Input: part model. Units: mm. Frame: model coordinates. A direction names the side the tool comes from. Round coordinates to 2 decimals unless told otherwise and drop trailing zeros. Loops run counter-clockwise (first coordinate to the right, second up) from the corner with the lowest first, then second, coordinate; pieces in that order, holes last.
1) Access query for faces 1 (the face through (1, 0.5, -3)), 2 (the face through (-3.787, 3.359, -0.841)), 3 (the face through (0.03, 1.11, 14.75)). Directions: +Z, -Z, +X, -X, +Y, -Y. A direction counts if a zero-diameter tool reaches every point of the face in a straight line with its end or side. Return the directions, or none.
2) First-contact query: pin 1 (5.5 mm diameter, centred on x = 1.5, z = 5.5, fed in from +Y); pin 2 (0.9 mm diameter, centred on x = 0, z = 15.5, fed in from -Y); pin 3 (4.5 mm diameter, centred on x = 0, z = 0, fed in from +Y); pin 4 (2 mm diameter, centred on x = 2, z = 7, fed in from +Y). Flat tips, straight axial feed; report the tip coordinate or a pass-through.
3) Section D-D, the plane y = 3.55. Return loops of the section in (x, z), and give its area (3 significant figures).
4) Section B-B, the plane z = 0. Return loops of the section in (x, y).
5) Ray query, line 1 along X through (y, z) = (0.4, 0.5); line 2 along X through (y, z) = (0.2, -0.75); line 3 along X through (y, z) = (1.3, 19). Return the intervals inside material, ascending.
6) Section A-A, the plane y = 1.9. Return loops of the section in (x, z).
7) Section C-C, the plane x = 0. State how many separate pieces and enclosed holes the cut face has, and give its area (3 significant figures).
8) Draft query along Z for faces 4 (the face through (-3, 4.5, 0)), 5 (the face through (0, 1.1, 20.6)), 6 (the face through (0.03, 1.11, 7.75)). Return one class per face: pulls with the +Z half, pulls with the -Z half, needs draft (parallel to the pull), parting line crosses it, or undercut.
from build123d import *

# Parameters (mm, degrees)
SKETCH1_R           = 2.5
SKETCH1_R_2         = 0.75
BOSS_EXTRUDE1_DEPTH = 2.25
SKETCH2_R           = 3.879501895
SKETCH2_R_2         = 2.5
BOSS_EXTRUDE2_DEPTH = 2.25
SKETCH3_R           = 2.5
SKETCH3_R_2         = 2.008527967
BOSS_EXTRUDE3_DEPTH = 1
SKETCH4_R           = 3.8
SKETCH4_R_2         = 3
CUT_EXTRUDE1_DEPTH  = 0.5
CUT_EXTRUDE2_DEPTH  = 22.766258291


with BuildPart() as part:
    # Sketch1 → Boss-Extrude1 (new body)
    with BuildSketch(Plane(origin=(0, 0, 0), x_dir=(1, 0, 0), z_dir=(0, 1, 0))):
        with BuildLine():
            Line((-1.6, 19), (-3.75, 3.885550154))
            ThreePointArc((-3.75, 3.885550154), (-5.4, 0), (-3.75, -3.885550154))
            Line((-3.75, -3.885550154), (-1.6, -19))
            ThreePointArc((-1.6, -19), (0, -20.6), (1.6, -19))
            Line((1.6, -19), (3.75, -3.885550154))
            ThreePointArc((3.75, -3.885550154), (5.4, 0), (3.75, 3.885550154))
            Line((3.75, 3.885550154), (1.6, 19))
            ThreePointArc((1.6, 19), (0, 20.6), (-1.6, 19))
        make_face()
        with Locations(Location((0, 0, 0), (0, 0, 270))):
            Circle(SKETCH1_R, mode=Mode.SUBTRACT)
        with Locations(Location((0, -19, 0), (0, 0, 270))):
            Circle(SKETCH1_R_2, mode=Mode.SUBTRACT)
        with Locations(Location((0, 19, 0), (0, 0, 270))):
            Circle(SKETCH1_R_2, mode=Mode.SUBTRACT)
        with Locations(Location((0, 15.5, 0), (0, 0, 270))):
            Circle(SKETCH1_R_2, mode=Mode.SUBTRACT)
        with Locations(Location((0, 12, 0), (0, 0, 270))):
            Circle(SKETCH1_R_2, mode=Mode.SUBTRACT)
        with Locations(Location((0, 8.5, 0), (0, 0, 270))):
            Circle(SKETCH1_R_2, mode=Mode.SUBTRACT)
        with Locations(Location((0, -15.5, 0), (0, 0, 270))):
            Circle(SKETCH1_R_2, mode=Mode.SUBTRACT)
        with Locations(Location((0, -12, 0), (0, 0, 270))):
            Circle(SKETCH1_R_2, mode=Mode.SUBTRACT)
        with Locations(Location((0, -8.5, 0), (0, 0, 270))):
            Circle(SKETCH1_R_2, mode=Mode.SUBTRACT)
    extrude(amount=BOSS_EXTRUDE1_DEPTH)

    # Sketch2 → Boss-Extrude2 (add)
    with BuildSketch(Plane(origin=(0, 2.25, 0), x_dir=(1, 0, 0), z_dir=(0, 1, 0))):
        with Locations(Location((0, 0, 0), (0, 0, 270))):
            Circle(SKETCH2_R)
        with Locations(Location((0, 0, 0), (0, 0, 270))):
            Circle(SKETCH2_R_2, mode=Mode.SUBTRACT)
    extrude(amount=BOSS_EXTRUDE2_DEPTH)

    # Sketch3 → Boss-Extrude3 (add)
    with BuildSketch(Plane.XZ):
        with Locations(Location((0, 0, 0), (0, 0, 270))):
            Circle(SKETCH3_R)
        with Locations(Location((0, 0, 0), (0, 0, 270))):
            Circle(SKETCH3_R_2, mode=Mode.SUBTRACT)
    extrude(amount=-BOSS_EXTRUDE3_DEPTH)

    # Sketch4 → Cut-Extrude1 (cut)
    with BuildSketch(Plane.XZ):
        with Locations(Location((0, 0, 0), (0, 0, 270))):
            Circle(SKETCH4_R)
        with Locations(Location((0, 0, 0), (0, 0, 270))):
            Circle(SKETCH4_R_2, mode=Mode.SUBTRACT)
    extrude(amount=-CUT_EXTRUDE1_DEPTH, mode=Mode.SUBTRACT)

    # Sketch5 → Cut-Extrude2 (cut, through all)
    with BuildSketch(Plane.XZ):
        with BuildLine():
            Line((-3.75, -3.885550154), (-1.6, -19))
            ThreePointArc((-1.6, -19), (0, -20.6), (1.6, -19))
            Line((1.6, -19), (3.75, -3.885550154))
            ThreePointArc((3.75, -3.885550154), (0, -5.4), (-3.75, -3.885550154))
        make_face()
    extrude(amount=-CUT_EXTRUDE2_DEPTH, mode=Mode.SUBTRACT)


solid = part.part
Final values:
1. face 1: -Y
1. face 2: +Y
1. face 3: +Y, -Y
2. pin 1: stops at y = 4.5
2. pin 2: passes through
2. pin 3: stops at y = 1
2. pin 4: stops at y = 2.25
3. outline: circle Ø7.76 at (0, 0); hole circle Ø5 at (0, 0)
3. area: 27.6 mm2
4. outline: (-5.4, 0) - (-3.8, 0) - (-3.8, 0.5) - (-3, 0.5) - (-3, 0) - (-2.01, 0) - (-2.01, 1) - (-2.5, 1) - (-2.5, 4.5) - (-3.88, 4.5) - (-3.88, 2.25) - (-5.4, 2.25) - close; (2.01, 0) - (3, 0) - (3, 0.5) - (3.8, 0.5) - (3.8, 0) - (5.4, 0) - (5.4, 2.25) - (3.88, 2.25) - (3.88, 4.5) - (2.5, 4.5) - (2.5, 1) - (2.01, 1) - close
5. line 1: x = -5.38 to -3.77, -2.96 to -1.95, 1.95 to 2.96, 3.77 to 5.38
5. line 2: x = -5.35 to -3.73, -2.9 to -1.86, 1.86 to 2.9, 3.73 to 5.35
5. line 3: x = -1.6 to -0.75, 0.75 to 1.6
6. outline: (-3.75, 3.89) arc R5.4 ccw (long way) to (3.75, 3.89) - (1.6, 19) arc R1.6 ccw to (-1.6, 19) - close; hole circle Ø5 at (0, 0); hole circle Ø1.5 at (0, 8.5); hole circle Ø1.5 at (0, 12); hole circle Ø1.5 at (0, 15.5); hole circle Ø1.5 at (0, 19)
7. separate pieces: 6
7. enclosed holes: 0
7. area: 40.1 mm2
8. face 4: needs draft
8. face 5: pulls with the +Z half
8. face 6: undercut
